Can you work these out from the model? Positions are in its coordinate system, mm. Round coordinates to 2 decimals unless told otherwise and drop trailing zeros. Loops run counter-clockwise (first coordinate to the right, second up) from the corner with the lowest first, then second, coordinate; pieces in that order, holes last. Notation, with made-up numbers: (-6.75, 88.5) -> (48.25, 88.5) arc R30 ccw to (48.25, 114.5) -> close; hole circle Ø5 at (-21, 53.5). An arc over 180 degrees is marked (long way). Use a Markdown table: item, result.
from build123d import *

# Parameters (mm, degrees)
F1_DEPTH = 0.2


# Not quite as in the source:
# - a feature names something its author has since deleted; it is built from what else it names


with BuildPart() as f1:
    # F0 (on Top) → F1 (new body)
    with BuildSketch(Plane.XY):
        Polygon((-110, -0.43), (-110, 0.43), (-110, 5), (-120, 5), (-120, -5), (-110, -5), align=None)
        with BuildLine():
            ThreePointArc((-4.981475685, -0.43), (-5, 0), (-4.981475685, 0.43))
            Line((-4.981475685, 0.43), (-110, 0.43))
            Line((-110, 0.43), (-110, -0.43))
            Line((-110, -0.43), (-4.981475685, -0.43))
        make_face()
        with BuildLine():
            ThreePointArc((-0.43, 4.981475685), (0, 5), (0.43, 4.981475685))
            Line((0.43, 4.981475685), (0.43, 90))
            Line((0.43, 90), (-0.43, 90))
            Line((-0.43, 90), (-0.43, 4.981475685))
        make_face()
        with BuildLine():
            ThreePointArc((4.981475685, 0.43), (4.9953667746, 0.2151994135), (5, 0))
            ThreePointArc((5, 0), (4.9953667746, -0.2151994135), (4.981475685, -0.43))
            Line((4.981475685, -0.43), (110, -0.43))
            Line((110, -0.43), (110, 0.43))
            Line((110, 0.43), (4.981475685, 0.43))
        make_face()
        with BuildLine():
            Line((0.43, -90), (0.43, -4.981475685))
            ThreePointArc((0.43, -4.981475685), (0, -5), (-0.43, -4.981475685))
            Line((-0.43, -4.981475685), (-0.43, -90))
            Line((-0.43, -90), (0.43, -90))
        make_face()
        Polygon((110, 5), (110, 0.43), (110, -0.43), (110, -5), (120, -5), (120, 5), align=None)
        Polygon((5, -90), (0.43, -90), (-0.43, -90), (-5, -90), (-5, -100), (5, -100), align=None)
        Polygon((-0.43, 90), (0.43, 90), (5, 90), (5, 100), (-5, 100), (-5, 90), align=None)
        with BuildLine():
            ThreePointArc((4.981475685, -0.43), (4.9953667746, -0.2151994135), (5, 0))
            ThreePointArc((5, 0), (4.9953667746, 0.2151994135), (4.981475685, 0.43))
            ThreePointArc((4.981475685, 0.43), (3.5355339059, 3.5355339059), (0.43, 4.981475685))
            ThreePointArc((0.43, 4.981475685), (0, 5), (-0.43, 4.981475685))
            ThreePointArc((-0.43, 4.981475685), (-3.5355339059, 3.5355339059), (-4.981475685, 0.43))
            ThreePointArc((-4.981475685, 0.43), (-5, 0), (-4.981475685, -0.43))
            ThreePointArc((-4.981475685, -0.43), (-3.5355339059, -3.5355339059), (-0.43, -4.981475685))
            ThreePointArc((-0.43, -4.981475685), (0, -5), (0.43, -4.981475685))
            ThreePointArc((0.43, -4.981475685), (3.5355339059, -3.5355339059), (4.981475685, -0.43))
        make_face()
    extrude(amount=F1_DEPTH)


solid = f1.part
1. Will this pin go through, and if not, where does the flat tip stop? pin 1 Ø12 at (x, y) = (7, -66.5) entering from -Z.
Answer sheet:
| item | result |
|---|---|
| pin 1 | passes through |
2. I want a section at B-B (x = -27). Please give me the cut outline in (y, z).
Answer sheet:
| item | result |
|---|---|
| outline | (-0.43, 0) -> (0.43, 0) -> (0.43, 0.2) -> (-0.43, 0.2) -> close |
3. I need wall thicknesses on line 1 (Y direction, x = -19.5, z = 0.1). Which ranges of the line are inside material? Lowest first, please.
Answer sheet:
| item | result |
|---|---|
| line 1 | y = -0.43 to 0.43 |
